Input: part model. Units: mm. Frame: model coordinates. Face numbers are marked on the shaded views. Round coordinates to 2 decimals unless told otherwise and drop trailing zeros. Loops run counter-clockwise (first coordinate to the right, second up) from the corner with the lowest first, then second, coordinate; pieces in that order, holes last. Notation, with made-up numbers: (-15.5, 14.25) -> (27.5, 14.25) arc R13 cw to (27.5, 31.25) -> close; hole circle Ø9 at (-36, 56.5). An arc over 180 degrees is marked (long way). Answer in a Markdown table with one row per item. Add a question column.
Q1. Section D-D, the plane z = -47.14. Output: boundary loops of the cut face in (x, y).
Q2. Section A-A, the plane z = -23.57. Output: boundary loops of the cut face in (x, y).
Q3. Pin query (flat end, axial travel): pin 1 (11 mm diameter, centred on x = 0, z = 0, fed in from -Y). Return the tip coordinate at first contact, or that it passes through.
Q4. Section C-C, the plane y = 8.25. Give the number of separate pieces and of enclosed holes in the cut face, and give its area (3 significant figures).
Q5. Mould query, pull axis Z, two halves, no side actions, for the marked faces 1 and 2. Classes: pulls with the +Z half, pulls with the -Z half, needs draft (parallel to the pull), parting line crosses it, or undercut.
Q6. Section B-B, the plane x = 47.14. Output: boundary loops of the cut face in (y, z), and give its area (3 significant figures).
Q7. Ray query, L1, parallel to X at y = 0.75, z = -68.5; L2, parallel to Z at x = 47.14, y = 6.75; L3, parallel to X at y = 8.35, z = 0. Return the intervals inside material, ascending. Write a range as from..to.
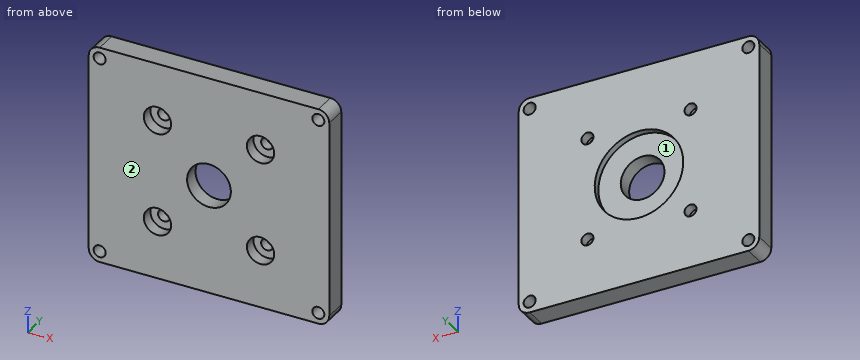
```python
from build123d import *

# Parameters (mm, degrees)
SKETCH2_W           = 110
SKETCH2_H           = 100
SKETCH2_R           = 2.75
BOSS_EXTRUDE1_DEPTH = 10
SKETCH3_R           = 10
CUT_EXTRUDE1_DEPTH  = 10
SKETCH4_R           = 20.25
CUT_EXTRUDE2_DEPTH  = 3
SKETCH5_R           = 6.25
CUT_EXTRUDE3_DEPTH  = 5.5
FILLET1_R           = 5


with BuildPart() as part:
    # Sketch2 → Boss-Extrude1 (new body)
    with BuildSketch(Plane(origin=(0, 0, 0), x_dir=(1, 0, 0), z_dir=(0, 1, 0))):
        with Locations((23.57, 23.57)):
            Rectangle(SKETCH2_W, SKETCH2_H)
        with Locations(Location((0, 47.14, 0), (0, 0, 270))):
            Circle(SKETCH2_R, mode=Mode.SUBTRACT)
        with Locations(Location((47.14, 47.14, 0), (0, 0, 270))):
            Circle(SKETCH2_R, mode=Mode.SUBTRACT)
        with Locations(Location((47.14, 0, 0), (0, 0, 270))):
            Circle(SKETCH2_R, mode=Mode.SUBTRACT)
        with Locations(Location((0, 0, 0), (0, 0, 270))):
            Circle(SKETCH2_R, mode=Mode.SUBTRACT)
        with Locations(Location((-26.43, 68.57, 0), (0, 0, 270))):
            Circle(SKETCH2_R, mode=Mode.SUBTRACT)
        with Locations(Location((73.57, 68.57, 0), (0, 0, 270))):
            Circle(SKETCH2_R, mode=Mode.SUBTRACT)
        with Locations(Location((73.57, -21.43, 0), (0, 0, 270))):
            Circle(SKETCH2_R, mode=Mode.SUBTRACT)
        with Locations(Location((-26.43, -21.43, 0), (0, 0, 270))):
            Circle(SKETCH2_R, mode=Mode.SUBTRACT)
    extrude(amount=BOSS_EXTRUDE1_DEPTH)

    # Sketch3 → Cut-Extrude1 (cut)
    with BuildSketch(Plane(origin=(0, 10, 0), x_dir=(1, 0, 0), z_dir=(0, 1, 0))):
        with Locations(Location((23.57, 23.57, 0), (0, 0, 270))):
            Circle(SKETCH3_R)
    extrude(amount=-CUT_EXTRUDE1_DEPTH, mode=Mode.SUBTRACT)

    # Sketch4 → Cut-Extrude2 (cut)
    with BuildSketch(Plane(origin=(0, 10, 0), x_dir=(1, 0, 0), z_dir=(0, 1, 0))):
        with Locations(Location((23.57, 23.57, 0), (0, 0, 270))):
            Circle(SKETCH4_R)
    extrude(amount=-CUT_EXTRUDE2_DEPTH, mode=Mode.SUBTRACT)

    # Sketch5 → Cut-Extrude3 (cut)
    with BuildSketch(Plane.XZ):
        with Locations(Location((0, 0, 0), (0, 0, 270))):
            Circle(SKETCH5_R)
        with Locations(Location((47.14, 0, 0), (0, 0, 270))):
            Circle(SKETCH5_R)
        with Locations(Location((47.14, -47.14, 0), (0, 0, 270))):
            Circle(SKETCH5_R)
        with Locations(Location((0, -47.14, 0), (0, 0, 270))):
            Circle(SKETCH5_R)
    extrude(amount=-CUT_EXTRUDE3_DEPTH, mode=Mode.SUBTRACT)

    # Fillet1
    fillet1_edges = [part.edges().sort_by_distance(p)[0] for p in [
        (78.57, 5, 26.43),
        (-31.43, 5, 26.43),
        (-31.43, 5, -73.57),
        (78.57, 5, -73.57),
    ]]
    fillet(fillet1_edges, radius=FILLET1_R)


solid = part.part
```
Answer block:
| question | item | result |
|---|---|---|
| 1 | outline | (-31.43, 0) -> (-6.25, 0) -> (-6.25, 5.5) -> (-2.75, 5.5) -> (-2.75, 10) -> (-31.43, 10) -> close; (2.75, 5.5) -> (6.25, 5.5) -> (6.25, 0) -> (40.89, 0) -> (40.89, 5.5) -> (44.39, 5.5) -> (44.39, 10) -> (2.75, 10) -> close; (49.89, 5.5) -> (53.39, 5.5) -> (53.39, 0) -> (78.57, 0) -> (78.57, 10) -> (49.89, 10) -> close |
| 2 | outline | (-31.43, 0) -> (13.57, 0) -> (13.57, 7) -> (3.32, 7) -> (3.32, 10) -> (-31.43, 10) -> close; (33.57, 0) -> (78.57, 0) -> (78.57, 10) -> (43.82, 10) -> (43.82, 7) -> (33.57, 7) -> close |
| 3 | pin 1 | y = 5.5 |
| 4 | separate pieces | 1 |
| 4 | enclosed holes | 9 |
| 4 | area | 9,500 mm^2 |
| 5 | face 1 | undercut |
| 5 | face 2 | needs draft |
| 6 | outline | (0, -73.57) -> (10, -73.57) -> (10, -49.89) -> (5.5, -49.89) -> (5.5, -53.39) -> (0, -53.39) -> close; (0, -40.89) -> (5.5, -40.89) -> (5.5, -44.39) -> (10, -44.39) -> (10, -2.75) -> (5.5, -2.75) -> (5.5, -6.25) -> (0, -6.25) -> close; (0, 6.25) -> (5.5, 6.25) -> (5.5, 2.75) -> (10, 2.75) -> (10, 26.43) -> (0, 26.43) -> close |
| 6 | area | 813 mm^2 |
| 7 | L1 | -31.43..-29.18, -23.68..70.82, 76.32..78.57 |
| 7 | L2 | -73.57..-49.89, -44.39..-2.75, 2.75..26.43 |
| 7 | L3 | -31.43..-2.75, 2.75..44.39, 49.89..78.57 |
